Check sheet for the modelled part. Datum: model origin and axes. Units: mm. A direction names the side the tool comes from. Coordinates: 2 decimals unless noted, no trailing zeros. Loops run counter-clockwise (first coordinate to the right, second up) from the corner with the lowest first, then second, coordinate; pieces in that order, holes last. Notation, with made-up numbers: (-35.75, 62) -> (-20.75, 62) arc R14 cw to (-20.75, 84) -> close; hole circle Ø6 at (-5.5, 1.5). An arc over 180 degrees is marked (long way). Use CSV: the item, a comma, the result in double quotes. Start each with the question number.
1. Gauge pin test, flat ends, axial feed: pin 1 (4 mm diameter, centred on x = -11, z = 3.5, fed in from -Y); pin 2 (2 mm diameter, centred on x = -1.5, y = 0, fed in from -Z); pin 3 (2.5 mm diameter, centred on x = 0, y = 7.1, fed in from -Z). Record the tip position at first contact, or that the pin passes through.
2. Set-up check for faces 4 (the face through (-21.21, -13.55, 2.46)), 5 (the face through (8.02, 36.12, -2.46)), 6 (the face through (4.918, -1.673, 4.014)): record each of +Z, -Z, +X, -X, +Y, -Y from which the full face is reachable in a straight line by a thin tool's end or side.
3. Sectioned sample at B-B, the plane y = -16.5. Record the cut outline in (x, z), and give its area (3 significant figures).
4. Thickness scan on L1, parallel to Y at x = 0, z = 2.2; L2, parallel to Y at x = 23.5, z = 2.5; L3, parallel to Z at x = 36, y = -16. Record the ranges inside material, lowest first.
5. Sectioned sample at C-C, the plane x = -33. Record the cut outline in (y, z), and give its area (3 significant figures).
6. Sectioned sample at A-A, the plane x = 22.65. Record the cut outline in (y, z).
7. Release check for a two-part mould opening along X. For faces 1 (the face through (-34.5, -14.3, -5)), 2 (the face through (1.48, 9.42, 4.01)), 3 (the face through (5.077, -38.668, -3.479)) record: pulls with the +X half, pulls with the -X half, needs draft (parallel to the pull), parting line crosses it, or undercut.
Autodesk Inventor part; units mm, degrees
ref_plane "YZ Plane" through (0, 0, 0) normal (1, 0, 0) x (0, 1, 0)
ref_plane "XZ Plane" through (0, 0, 0) normal (0, 1, 0) x (-1, 0, 0)
ref_plane "XY Plane" through (0, 0, 0) normal (0, 0, 1) x (1, 0, 0)
sketch "Szkic1" plane through (0, 0, 0) normal (0, 0, 1) x (1, 0, 0)
  circle A0 centre (0, 0) radius 10.75
  circle A1 centre (0, 0) radius 11.25
  circle A2 centre (0, 0) radius 43
  dimension "d0" = 21.5
  dimension "d1" = 0.5
  dimension "d2" = 86
extrude "Wyciągnięcie proste1" add sketch "Szkic1" along normal blind 10 contours A0 | A1 | A2
sketch "Szkic2" plane through (0, 0, 10) normal (0, 0, 1) x (1, 0, 0)
  circle A0 centre (0, 0) radius 3.5
  point P0 (7.1, 0)
  point P1 (0, 7.1)
  point P2 (-7.1, 0)
  point P3 (0, -7.1)
  dimension "d5" = 7.1
  dimension "d6" = 7.1
  dimension "d7" = 7.1
  dimension "d8" = 7.1
  dimension "d9" = 7
hole "Otwór1" at (7.1, 0, 10) at (0, 7.1, 10) at (-7.1, 0, 10) at (0, -7.1, 10) direction (0, 0, -1) diameter 1.567 end through all
sketch "Szkic3" plane through (0, 0, 0) normal (0, 0, -1) x (-1, 0, 0)
  circle A0 centre (0, 0) radius 11.5
  dimension "d17" = 23
extrude "Wyciągnięcie proste2" cut sketch "Szkic3" against normal blind 2
sketch "Szkic4" plane through (0, 0, 2) normal (0, 0, -1) x (-1, 0, 0)
  circle A0 centre (0, 0) radius 3.5
  dimension "d20" = 7
extrude "Wyciągnięcie proste3" cut sketch "Szkic4" against normal blind 1
sketch "Szkic5" plane through (0, 0, 10) normal (0, 0, 1) x (1, 0, 0)
  circle A0 centre (-7.1, 0) radius 0.7835
  circle A1 centre (7.1, 0) radius 0.7835
  circle A2 centre (0, 7.1) radius 0.7835
  circle A3 centre (0, -7.1) radius 0.7835
  circle A4 centre (0, 0) radius 43
extrude "Wyciągnięcie proste4" cut sketch "Szkic5" against normal blind 5
sketch "Szkic6" plane through (0, 0, 5) normal (0, 0, 1) x (1, 0, 0)
  circle A0 centre (0, -7.1) radius 0.7835
  circle A1 centre (7.1, 0) radius 0.7835
  circle A2 centre (-7.1, 0) radius 0.7835
  circle A3 centre (0, 7.1) radius 0.7835
  circle A4 centre (0, -7.1) radius 2.75
  circle A5 centre (-7.1, 0) radius 0.7835
  circle A6 centre (-7.1, 0) radius 2.75
  circle A7 centre (0, 7.1) radius 2.75
  circle A8 centre (7.1, 0) radius 0.7835
  circle A9 centre (7.1, 0) radius 2.75
  point P0 (0, 0)
  dimension "d25" = 5.5
  dimension "d26" = 5.5
  dimension "d27" = 5.5
  dimension "d28" = 5.5
extrude "Wyciągnięcie proste5" cut sketch "Szkic6" against normal blind 2 contours A3 | A4 | A6 | A7 | A9
sketch "Szkic9" plane through (0, 0, 0) normal (0, 0, -1) x (-1, 0, 0)
  circle A0 centre (0, 0) radius 11.5
  circle A1 centre (0, 0) radius 43
  circle A2 centre (0, 0) radius 37
  dimension "d36" = 6
extrude "Wyciągnięcie proste7" add sketch "Szkic9" along normal blind 2 contours A1
sketch "Szkic10" plane through (0, 0, -2) normal (0, 0, -1) x (-1, 0, 0)
  circle A0 centre (0, 0) radius 43
  circle A1 centre (0, 0) radius 37
  circle A2 centre (0, 0) radius 39
  dimension "d39" = 2
extrude "Wyciągnięcie proste8" add sketch "Szkic10" along normal blind 3 contours A2
sketch "Szkic12" plane through (0, 0, 5) normal (0, 0, 1) x (1, 0, 0)
  line L0 (-30.65, -20.8055) -> (30.65, -20.8055)
  line L1 (30.65, -20.8055) -> (30.65, 20.8055)
  line L2 (30.65, 20.8055) -> (-30.65, 20.8055)
  line L3 (-30.65, 20.8055) -> (-30.65, -20.8055)
  line L4 (-30.65, -20.8055) -> (30.65, 20.8055) construction
  line L5 (30.65, -20.8055) -> (-30.65, 20.8055) construction
  point P0 (0, 0)
  point P1 (-22.65, 12.8055)
  point P2 (-22.65, -12.8055)
  point P3 (22.65, 12.8055)
  point P4 (22.65, -12.8055)
  dimension "d59" = 61.3
  dimension "d60" = 41.611
  dimension "d61" = 8
  dimension "d62" = 8
  dimension "d63" = 8
  dimension "d64" = 8
  dimension "d65" = 8
  dimension "d66" = 8
  dimension "d67" = 8
  dimension "d68" = 8
hole "Otwór3" at (-22.65, 12.8055, 5) at (-22.65, -12.8055, 5) at (22.65, 12.8055, 5) at (22.65, -12.8055, 5) direction (0, 0, -1) diameter 3.242 end through all
properties part number "Podstawa2_Drukowanie 3D"
Completed:
1,pin 1,"y = -42.05"
1,pin 2,"z = 3"
1,pin 3,"z = 2"
2,face 4,"+Z, -Z"
2,face 5,"-Z"
2,face 6,"+Z"
3,outline,"(-39.71, -2) -> (-35.34, -2) -> (-35.34, -5) -> (-33.12, -5) -> (-33.12, 0) -> (33.12, 0) -> (33.12, -5) -> (35.34, -5) -> (35.34, -2) -> (39.71, -2) -> (39.71, 5) -> (-39.71, 5) -> close"
3,area,"437 mm²"
4,L1,"-43 to -7.88, -6.32 to -3.5, 3.5 to 6.32, 7.88 to 43"
4,L2,"-36.01 to -14.19, -11.43 to 11.43, 14.19 to 36.01"
4,L3,"-2 to 5"
5,outline,"(-27.57, -2) -> (-20.78, -2) -> (-20.78, -5) -> (-16.73, -5) -> (-16.73, 0) -> (16.73, 0) -> (16.73, -5) -> (20.78, -5) -> (20.78, -2) -> (27.57, -2) -> (27.57, 5) -> (-27.57, 5) -> close"
5,area,"343 mm²"
6,outline,"(-36.55, -2) -> (-31.75, -2) -> (-31.75, -5) -> (-29.26, -5) -> (-29.26, 0) -> (-14.43, 0) -> (-14.43, 5) -> (-36.55, 5) -> close; (-11.18, 0) -> (11.18, 0) -> (11.18, 5) -> (-11.18, 5) -> close; (14.43, 0) -> (29.26, 0) -> (29.26, -5) -> (31.75, -5) -> (31.75, -2) -> (36.55, -2) -> (36.55, 5) -> (14.43, 5) -> close"
7,face 1,"needs draft"
7,face 2,"undercut"
7,face 3,"parting line crosses it"
